```python
from build123d import *

# Parameters (mm, degrees)
EXTRUDE_1_DEPTH          = 5
CUT_EXTRUDE_1_DEPTH      = 13.247448714
CUT_EXTRUDE_1_DEPTH_BACK = 13.247448714
SKETCH_2_R               = 1.5
CUT_EXTRUDE_2_DEPTH      = 13.247448714
CUT_EXTRUDE_2_DEPTH_BACK = 13.247448714
SKETCH_3_R               = 1.5


with BuildPart() as part:
    # 草图1 → 凸台-拉伸1 (new, symmetric)
    with BuildSketch(Plane.XY):
        Polygon((-5, 5), (-5, -5), (5, -5), align=None)
    extrude(amount=EXTRUDE_1_DEPTH, both=True)

    # 草图2 → 切除-拉伸1 (cut, two sides: drawn at the far end of the back side and taken through both)
    with BuildSketch(Plane.ZY.offset(5).offset(-CUT_EXTRUDE_1_DEPTH_BACK)):
        with Locations(Location((0, 0, 0), (0, 0, 90))):
            Circle(SKETCH_2_R)
    extrude(amount=CUT_EXTRUDE_1_DEPTH + CUT_EXTRUDE_1_DEPTH_BACK, mode=Mode.SUBTRACT)

    # 草图3 → 切除-拉伸2 (cut, two sides: drawn at the far end of the back side and taken through both)
    with BuildSketch(Plane.XZ.offset(5).offset(-CUT_EXTRUDE_2_DEPTH_BACK)):
        with Locations(Location((0, 0, 0), (0, 0, 90))):
            Circle(SKETCH_3_R)
    extrude(amount=CUT_EXTRUDE_2_DEPTH + CUT_EXTRUDE_2_DEPTH_BACK, mode=Mode.SUBTRACT)


solid = part.part
```
Model file for the job. Use its own axes, mm. Round coordinates to 2 decimals unless told otherwise and drop trailing zeros. Write each loop counter-clockwise with the first axis right and the second up, starting at its lowest first coordinate (ties: lowest second). Pieces come first, ordered by that corner, then holes. Notation, with made-up numbers: (11, -31) -> (55, -31) arc R14 cw to (55, -8) -> close; hole circle Ø5 at (-22, 8). An arc over 180 degrees is marked (long way). Answer as CSV lines item,"result".
1. Pin check, flat tips, straight feed: pin 1 Ø1 at (x, z) = (-0.5, -1.5) entering from +Y; pin 2 Ø1 at (x, z) = (-2, 0.5) entering from +Y; pin 3 Ø4 at (x, z) = (0, 0) entering from +Y. Stop position of each tip, or through.
Resolved:
pin 1,"y = 1"
pin 2,"y = 2.5"
pin 3,"y = 2"
2. Slice it at A-A, the plane x = -3.25. List the corners of the cut face in (y, z), plus the area to 3 significant figures.
Resolved:
outline,"(-5, -5) -> (3.25, -5) -> (3.25, 5) -> (-5, 5) -> close; hole circle Ø3 at (0, 0)"
area,"75.4 mm²"
3. Mould opens along Y. For faces 1 (the face through (-1.2, -5, 1.2)), 2 (the face through (-2, -2, 5)), 3 (the face through (-3.02, -1.5, -0.07)), 4 (the face through (1.2, -1.2, 1.2)) say: +Y half, -Y half, draft (parallel to the pull), parting line (faces both ways), or undercut.
Resolved:
face 1,"-Y half"
face 2,"draft"
face 3,"undercut"
face 4,"+Y half"
4. Drill centre lines: line 1 (Z direction, x = 0, y = -0.95); line 2 (Y direction, x = 0, z = -2.5); line 3 (X direction, y = -2.5, z = -0.5). Where is each one in solid material? Low to high.
Resolved:
line 1,"-5 to -1.5, 1.5 to 5"
line 2,"-5 to 0"
line 3,"-5 to -1.41, 1.41 to 2.5"
5. Slice it at C-C, the plane y = -1. List the corners of the cut face in (x, z), plus the area to 3 significant figures.
Resolved:
outline,"(-5, -5) -> (1, -5) -> (1, -1.12) arc R1.5 cw to (-1, -1.12) -> (-5, -1.12) -> close; (-5, 1.12) -> (-1, 1.12) arc R1.5 cw to (1, 1.12) -> (1, 5) -> (-5, 5) -> close"
area,"45.5 mm²"
6. Slice it at D-D, the plane z = 3. List the corners of the cut face in (x, y).
Resolved:
outline,"(-5, -5) -> (5, -5) -> (-5, 5) -> close"
7. Slice it at B-B, the plane z = 0. List the corners of the cut face in (x, y), plus the area to 3 significant figures.
Resolved:
outline,"(-5, -5) -> (-1.5, -5) -> (-1.5, -1.5) -> (-5, -1.5) -> close; (-5, 1.5) -> (-1.5, 1.5) -> (-5, 5) -> close; (1.5, -5) -> (5, -5) -> (1.5, -1.5) -> close"
area,"24.5 mm²"
